Can you work these out from the model? Positions are in its coordinate system, mm. Face numbers are marked on the shaded views. Coordinates: 2 decimals unless noted, no trailing zeros. Loops run counter-clockwise (first coordinate to the right, second up) from the corner with the lowest first, then second, coordinate; pieces in that order, holes last. Notation, with made-up numbers: (55, -2.5) - (97, -2.5) arc R28 cw to (97, 35.5) - close; hole circle Ø1 at (-32, 59). An arc over 180 degrees is marked (long way). Put each result on its own line as item: value. Start each with the question number.
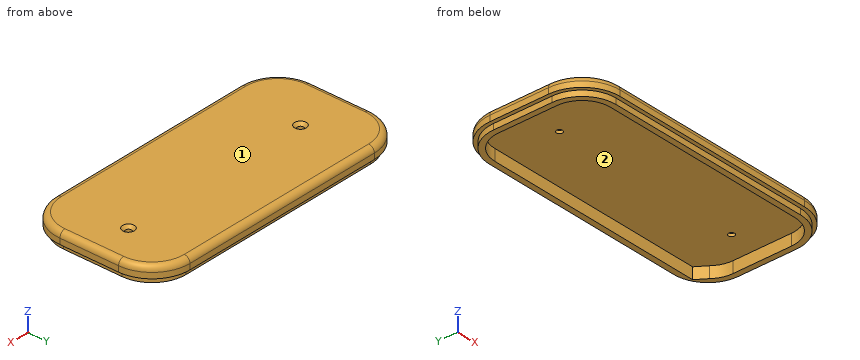
from build123d import *

# Parameters (mm, degrees)
BOSS_EXTRUDE1_DEPTH = 3
BOSS_EXTRUDE2_START = 3
BOSS_EXTRUDE2_DEPTH = 3
FILLET1_R           = 3
BOSS_EXTRUDE3_START = 6
BOSS_EXTRUDE3_DEPTH = 6
SKETCH4_R           = 1.6
CUT_EXTRUDE1_DEPTH  = 3
CHAMFER1_SIZE       = 1.5
CUT_EXTRUDE2_DEPTH  = 6


with BuildPart() as part:
    # Sketch1 → Boss-Extrude1 (new body)
    with BuildSketch(Plane.XY):
        with BuildLine():
            Line((67.5, -46), (67.5, -15))
            ThreePointArc((67.5, -15), (61.642135624, -0.857864376), (47.5, 5))
            Line((47.5, 5), (-62.5, 5))
            ThreePointArc((-62.5, 5), (-76.642135624, -0.857864376), (-82.5, -15))
            Line((-82.5, -15), (-82.5, -46))
            ThreePointArc((-82.5, -46), (-76.642135624, -60.142135624), (-62.5, -66))
            Line((-62.5, -66), (47.5, -66))
            ThreePointArc((47.5, -66), (61.642135624, -60.142135624), (67.5, -46))
        make_face()
    extrude(amount=BOSS_EXTRUDE1_DEPTH)

    # Sketch2 → Boss-Extrude2 (add)
    with BuildSketch(Plane(origin=(0, 0, 0), x_dir=(-1, 0, 0), z_dir=(0, 0, -1)).offset(BOSS_EXTRUDE2_START)):
        with BuildLine():
            Line((-47.5, -66), (62.5, -66))
            ThreePointArc((62.5, -66), (76.642135624, -60.142135624), (82.5, -46))
            Line((82.5, -46), (82.5, -15))
            ThreePointArc((82.5, -15), (76.642135624, -0.857864376), (62.5, 5))
            Line((62.5, 5), (-47.5, 5))
            ThreePointArc((-47.5, 5), (-61.642135624, -0.857864376), (-67.5, -15))
            Line((-67.5, -15), (-67.5, -46))
            ThreePointArc((-67.5, -46), (-61.642135624, -60.142135624), (-47.5, -66))
        make_face()
        with BuildLine():
            Line((-47.5, -64), (62.5, -64))
            ThreePointArc((62.5, -64), (75.227922061, -58.727922061), (80.5, -46))
            Line((80.5, -46), (80.5, -15))
            ThreePointArc((80.5, -15), (75.227922061, -2.272077939), (62.5, 3))
            Line((62.5, 3), (-47.5, 3))
            ThreePointArc((-47.5, 3), (-60.227922061, -2.272077939), (-65.5, -15))
            Line((-65.5, -15), (-65.5, -46))
            ThreePointArc((-65.5, -46), (-60.227922061, -58.727922061), (-47.5, -64))
        make_face(mode=Mode.SUBTRACT)
    extrude(amount=-BOSS_EXTRUDE2_DEPTH)

    # Fillet1
    fillet1_edges = [part.edges().sort_by_distance(p)[0] for p in [
        (61.642135624, -0.857864376, 3),
        (-7.5, 5, 3),
        (-76.642135624, -0.857864376, 3),
        (-82.5, -30.5, 3),
        (-76.642135624, -60.142135624, 3),
        (-7.5, -66, 3),
        (61.642135624, -60.142135624, 3),
        (67.5, -30.5, 3),
    ]]
    fillet(fillet1_edges, radius=FILLET1_R)

    # Sketch3 → Boss-Extrude3 (add)
    with BuildSketch(Plane(origin=(0, 0, 0), x_dir=(-1, 0, 0), z_dir=(0, 0, -1)).offset(BOSS_EXTRUDE3_START)):
        with BuildLine():
            Line((-65.5, -15), (-65.5, -46))
            ThreePointArc((-65.5, -46), (-60.227922061, -58.727922061), (-47.5, -64))
            Line((-47.5, -64), (62.5, -64))
            ThreePointArc((62.5, -64), (75.227922061, -58.727922061), (80.5, -46))
            Line((80.5, -46), (80.5, -15))
            ThreePointArc((80.5, -15), (75.227922061, -2.272077939), (62.5, 3))
            Line((62.5, 3), (-47.5, 3))
            ThreePointArc((-47.5, 3), (-60.227922061, -2.272077939), (-65.5, -15))
        make_face()
        with BuildLine():
            Line((-62.5, -15), (-62.5, -46))
            ThreePointArc((-62.5, -46), (-58.106601718, -56.606601718), (-47.5, -61))
            Line((-47.5, -61), (62.5, -61))
            ThreePointArc((62.5, -61), (73.106601718, -56.606601718), (77.5, -46))
            Line((77.5, -46), (77.5, -15))
            ThreePointArc((77.5, -15), (73.106601718, -4.393398282), (62.5, 0))
            Line((62.5, 0), (-47.5, 0))
            ThreePointArc((-47.5, 0), (-58.106601718, -4.393398282), (-62.5, -15))
        make_face(mode=Mode.SUBTRACT)
    extrude(amount=-BOSS_EXTRUDE3_DEPTH)

    # Sketch4 → Cut-Extrude1 (cut)
    with BuildSketch(Plane(origin=(0, 0, 0), x_dir=(-1, 0, 0), z_dir=(0, 0, -1))):
        with Locations((-47.5, -27.5)):
            Circle(SKETCH4_R)
        with Locations((55.1, -27.5)):
            Circle(SKETCH4_R)
    extrude(amount=-CUT_EXTRUDE1_DEPTH, mode=Mode.SUBTRACT)

    # Chamfer1
    chamfer1_edges = [part.edges().sort_by_distance(p)[0] for p in [
        (49.1, -27.5, 3),
        (-53.5, -27.5, 3),
    ]]
    chamfer(chamfer1_edges, length=CHAMFER1_SIZE)

    # Sketch5 → Cut-Extrude2 (cut)
    with BuildSketch(Plane(origin=(0, 0, -6), x_dir=(-1, 0, 0), z_dir=(0, 0, -1))):
        Polygon((-44.433816438, 0), (-55.308762061, 0), (-60.500068825, -7.51680479), align=None)
    extrude(amount=-CUT_EXTRUDE2_DEPTH, mode=Mode.SUBTRACT)


solid = part.part
Q1. We'd pull the mould along X, two halves only. Please class the marked faces 1 and 2: released by +X, released by -X, zero draft, split by the parting line, or undercut.
Q2. I want a section at D-D on y = -19. List the corners of the cut face in (x, z) for me.
Q3. I want a section at C-C on x = -55.1. List the corners of the cut face in (y, z) for me.
Q4. I want a section at B-B on z = -4.5. List the corners of the cut face in (x, y) for me.
Q5. I want a section at A-A on y = -27.5. List the corners of the cut face in (x, z) for me.
Q6. Will these pins go through, and if not, where does the flat tip stop? pin 1 (1.5 mm diameter, centred on y = -25, z = -5, fed in from -X); pin 2 (3 mm diameter, centred on y = -29, z = -3.5, fed in from -X); pin 3 (1 mm diameter, centred on x = -13, z = -5, fed in from +Y); pin 4 (0.9 mm diameter, centred on x = 6, z = -4, fed in from -Y).
Q7. Please list where these lines run through material, in increasing order: line 1 along X through (y, z) = (-39.5, -5.5); line 2 along Y through (x, z) = (-15.5, -0.75); line 3 along Y through (x, z) = (26, -4). Write a range as [from, to].
Calculated:
1. face 1: zero draft
1. face 2: undercut
2. outline: (-82.5, -3) - (-80.5, -3) - (-80.5, -6) - (-77.5, -6) - (-77.5, 0) - (62.5, 0) - (62.5, -6) - (65.5, -6) - (65.5, -3) - (67.5, -3) - (67.5, 0) arc R3 ccw to (64.5, 3) - (-79.5, 3) arc R3 ccw to (-82.5, 0) - close
3. outline: (-66, -3) - (-64, -3) - (-64, -6) - (-61, -6) - (-61, 0) - (-29.1, 0) - (-29.1, 1.5) - (-30.6, 3) - (-63, 3) arc R3 ccw to (-66, 0) - close; (-25.9, 0) - (0, 0) - (0, -6) - (3, -6) - (3, -3) - (5, -3) - (5, 0) arc R3 ccw to (2, 3) - (-24.4, 3) - (-25.9, 1.5) - close
4. outline: (-80.5, -46) arc R18 ccw to (-62.5, -64) - (47.5, -64) arc R18 ccw to (65.5, -46) - (65.5, -15) arc R18 ccw to (47.5, 3) - (-62.5, 3) arc R18 ccw to (-80.5, -15) - close; hole (-77.5, -46) arc R15 ccw to (-62.5, -61) - (47.5, -61) arc R15 ccw to (62.5, -46) - (62.5, -15) arc R15 ccw to (59.1, -5.49) - (55.31, 0) - (-62.5, 0) arc R15 ccw to (-77.5, -15) - close
5. outline: (-82.5, -3) - (-80.5, -3) - (-80.5, -6) - (-77.5, -6) - (-77.5, 0) - (-56.7, 0) - (-56.7, 1.5) - (-58.2, 3) - (-79.5, 3) arc R3 ccw to (-82.5, 0) - close; (-53.5, 0) - (45.9, 0) - (45.9, 1.5) - (44.4, 3) - (-52, 3) - (-53.5, 1.5) - close; (49.1, 0) - (62.5, 0) - (62.5, -6) - (65.5, -6) - (65.5, -3) - (67.5, -3) - (67.5, 0) arc R3 ccw to (64.5, 3) - (50.6, 3) - (49.1, 1.5) - close
6. pin 1: x = -80.5
6. pin 2: x = -82.5
6. pin 3: y = 3
6. pin 4: y = -64
7. line 1: [-80.5, -77.5], [62.5, 65.5]
7. line 2: [-66, -61], [0, 5]
7. line 3: [-64, -61], [0, 3]
